from build123d import *

# Parameters (mm, degrees)
SKETCH1_W           = 74.75
SKETCH1_H           = 40
BOSS_EXTRUDE1_DEPTH = 3
SKETCH2_W           = 2.25
SKETCH2_H           = 10.5
CUT_EXTRUDE1_DEPTH  = 85.832555661
FILLET2_R           = 2.25
FILLET1_R           = 2.25
BOSS_EXTRUDE4_DEPTH = 3.7
SKETCH7_W           = 68.5
SKETCH7_H           = 35.5
OLED_RECESS_DEPTH   = 1.5
SKETCH9_R           = 1.7
SKETCH9_W           = 38
SKETCH9_H           = 18
CUT_EXTRUDE5_DEPTH  = 85.860193848


with BuildPart() as part:
    # Sketch1 → Boss-Extrude1 (new body)
    with BuildSketch(Plane.XY):
        with Locations((37.375, 20)):
            Rectangle(SKETCH1_W, SKETCH1_H)
    extrude(amount=BOSS_EXTRUDE1_DEPTH)

    # Sketch2 → Cut-Extrude1 (cut, through all)
    with BuildSketch(Plane.XY.offset(3)):
        with Locations((1.125, 20)):
            Rectangle(SKETCH2_W, SKETCH2_H)
    extrude(amount=-CUT_EXTRUDE1_DEPTH, mode=Mode.SUBTRACT)

    # Fillet2
    fillet2_edges = [part.edges().sort_by_distance(p)[0] for p in [
        (0, 14.75, 1.5),
        (0, 25.25, 1.5),
    ]]
    fillet(fillet2_edges, radius=FILLET2_R - 0.0001)  # a hair under: the kernel refuses the full size

    # Fillet1
    fillet1_edges = [part.edges().sort_by_distance(p)[0] for p in [
        (0, 40, 1.5),
        (0, 0, 1.5),
    ]]
    fillet(fillet1_edges, radius=FILLET1_R)

    # Sketch6 → Boss-Extrude4 (add)
    with BuildSketch(Plane.XY.offset(3)):
        with BuildLine():
            Line((1.25, 25.484435563), (1.25, 14.515564437))
            ThreePointArc((1.25, 14.515564437), (1.736443763, 14.69060722), (2.25, 14.75))
            Line((2.25, 14.75), (2.25, 25.25))
            ThreePointArc((2.25, 25.25), (1.736443763, 25.30939278), (1.25, 25.484435563))
        make_face()
    extrude(amount=-BOSS_EXTRUDE4_DEPTH)

    # Sketch7 → oled-recess (cut)
    with BuildSketch(Plane(origin=(0, 0, 0), x_dir=(-1, 0, 0), z_dir=(0, 0, -1))):
        with Locations((-38.25, 20)):
            Rectangle(SKETCH7_W, SKETCH7_H)
    extrude(amount=-OLED_RECESS_DEPTH, mode=Mode.SUBTRACT)

    # Sketch9 → Cut-Extrude5 (cut, through all)
    with BuildSketch(Plane.XY.offset(3)):
        with Locations((6, 34)):
            Circle(SKETCH9_R)
        with Locations((69, 34)):
            Circle(SKETCH9_R)
        with Locations((6, 6)):
            Circle(SKETCH9_R)
        with Locations((69, 6)):
            Circle(SKETCH9_R)
        with Locations((37.5, 20)):
            Rectangle(SKETCH9_W, SKETCH9_H)
        with BuildLine():
            Line((8, 28.5), (8, 23.5))
            Line((8, 23.5), (8.3, 23.5))
            Line((8.3, 23.5), (8.3, 28.5))
            ThreePointArc((8.3, 28.5), (12, 32.2), (15.7, 28.5))
            Line((15.7, 28.5), (15.7, 23.5))
            Line((15.7, 23.5), (16, 23.5))
            Line((16, 23.5), (16, 28.5))
            ThreePointArc((16, 28.5), (12, 32.5), (8, 28.5))
        make_face()
        with BuildLine():
            Line((15.7, 16.5), (16, 16.5))
            Line((16, 16.5), (16, 11.5))
            ThreePointArc((16, 11.5), (12, 7.5), (8, 11.5))
            Line((8, 11.5), (8, 16.5))
            Line((8, 16.5), (8.3, 16.5))
            Line((8.3, 16.5), (8.3, 11.5))
            ThreePointArc((8.3, 11.5), (12, 7.8), (15.7, 11.5))
            Line((15.7, 11.5), (15.7, 16.5))
        make_face()
    extrude(amount=-CUT_EXTRUDE5_DEPTH, mode=Mode.SUBTRACT)


solid = part.part
Work out the finished part from the listing and answer in its coordinate system (mm). A direction names the side the tool comes from. Give positions to 0.01 mm unless a question says otherwise; leave off trailing zeros. Order: outer loops, then holes, each group sorted by start corner. A loop starts at its lowest first (then second) coordinate and runs counter-clockwise, first axis right, second up. Notation, with made-up numbers: (21, 28.5) -> (40, 28.5) arc R27 cw to (40, 67.5) -> close; hole circle Ø11 at (20.25, 2). An arc over 180 degrees is marked (long way). One line per item, written item: value.
Item 1: A tool of negligible diameter and unlimited length cuts with its end or side. For faces 1 (the cylindrical face through (0.68, 39.36, 1.52)), 2 (the flat face through (74.75, 20, 1)), 3 (the flat face through (39, 37.75, 1)), 4 (the flat face through (16, 14, 2)), 5 (the flat face through (1.25, 20, 1)), from which of +Z, -Z, +X, -X, +Y, -Y can it reach the whole face along a straight path? Write none if from no direction.
Answer sheet:
face 1: +Z, -Z, -X, +Y
face 2: +Z, -Z, +X, +Y, -Y
face 3: -Z
face 4: +Z, -Z
face 5: +Z, -Z, -X
Item 2: Find section A-A, the plane y = 34. Give the vertices of the cut face in (x, z).
Answer sheet:
outline: (0, 0) -> (4, 0) -> (4, 1.5) -> (4.3, 1.5) -> (4.3, 3) -> (0, 3) -> close; (7.7, 1.5) -> (67.3, 1.5) -> (67.3, 3) -> (7.7, 3) -> close; (70.7, 1.5) -> (72.5, 1.5) -> (72.5, 0) -> (74.75, 0) -> (74.75, 3) -> (70.7, 3) -> close
Item 3: Flat-ended cylindrical pins translate along their axes: P1, Ø4.5, axis at x = 69, y = 6, coming from the -Z side; P2, Ø1.8, axis at y = 20.5, z = 1, coming from the -X side. Find the tip coordinate at first contact, or state that the pin passes through.
Answer sheet:
P1: z = 1.5
P2: x = 1.25
Item 4: Find section D-D, the plane x = 22.5. Give the vertices of the cut face in (y, z), plus the area to 4 significant figures.
Answer sheet:
outline: (0, 0) -> (2.25, 0) -> (2.25, 1.5) -> (11, 1.5) -> (11, 3) -> (0, 3) -> close; (29, 1.5) -> (37.75, 1.5) -> (37.75, 0) -> (40, 0) -> (40, 3) -> (29, 3) -> close
area: 39.75 mm²
Item 5: Straight lines are drawn through the part: probe 1 along Y at (x, z) = (69, 2.3); probe 2 along Y at (x, z) = (34, 1.65); probe 3 along X at (y, z) = (36, 0.9). For each, find the intervals that lie inside material, in ascending order.
Answer sheet:
probe 1: 0 to 4.3, 7.7 to 32.3, 35.7 to 40
probe 2: 0 to 11, 29 to 40
probe 3: 0 to 4, 72.5 to 74.75
Item 6: Determine the mould class of faces 6 (the flat face through (8, 14, 2)), 7 (the flat face through (38, 0, 1)), 8 (the cylindrical face through (0.33, 13.67, 1.48)) for opening direction X: released by +X, released by -X, zero draft, split by the parting line, or undercut.
Answer sheet:
face 6: undercut
face 7: zero draft
face 8: released by -X
Item 7: Find section B-B, the plane x = 12. Give the vertices of the cut face in (y, z), plus the area to 4 significant figures.
Answer sheet:
outline: (0, 0) -> (2.25, 0) -> (2.25, 1.5) -> (7.5, 1.5) -> (7.5, 3) -> (0, 3) -> close; (7.8, 1.5) -> (32.2, 1.5) -> (32.2, 3) -> (7.8, 3) -> close; (32.5, 1.5) -> (37.75, 1.5) -> (37.75, 0) -> (40, 0) -> (40, 3) -> (32.5, 3) -> close
area: 65.85 mm²
Item 8: Find section C-C, the plane z = 0.85. Give the vertices of the cut face in (x, y), plus the area to 3 significant figures.
Answer sheet:
outline: (0, 2.25) arc R2.25 ccw to (2.25, 0) -> (74.75, 0) -> (74.75, 40) -> (2.25, 40) arc R2.25 ccw to (0, 37.75) -> (0, 27.5) arc R2.25 ccw to (1.25, 25.48) -> (1.25, 14.52) arc R2.25 ccw to (0, 12.5) -> close; hole (4, 2.25) -> (72.5, 2.25) -> (72.5, 37.75) -> (4, 37.75) -> close
area: 541 mm²
